Verification items for the finished model (mm, model axes). Give positions to 0.01 mm unless a question says otherwise; leave off trailing zeros. Write each loop counter-clockwise with the first axis right and the second up, starting at its lowest first coordinate (ties: lowest second). Pieces come first, ordered by that corner, then holes.
from build123d import *

# Parameters (mm, degrees)
SKETCH_1_W          = 8
SKETCH_1_H          = 8
EXTRUDE_1_DEPTH     = 20
SKETCH_3_R          = 1.5
CUT_EXTRUDE_1_DEPTH = 23.978250586
SKETCH_5_R          = 1.5
CUT_EXTRUDE_2_DEPTH = 23.978250586


with BuildPart() as part:
    # 草图1 → 凸台-拉伸1 (new body)
    with BuildSketch(Plane(origin=(0, 0, 0), x_dir=(0, 0, -1), z_dir=(1, 0, 0))):
        with Locations((4, 4)):
            Rectangle(SKETCH_1_W, SKETCH_1_H)
    extrude(amount=EXTRUDE_1_DEPTH)

    # 草图3 → 切除-拉伸1 (cut, through all)
    with BuildSketch(Plane.XY):
        with Locations((4, 4)):
            Circle(SKETCH_3_R)
        with Locations((16, 4)):
            Circle(SKETCH_3_R)
    extrude(amount=-CUT_EXTRUDE_1_DEPTH, mode=Mode.SUBTRACT)

    # 草图5 → 切除-拉伸2 (cut, through all)
    with BuildSketch(Plane(origin=(0, 8, 0), x_dir=(1, 0, 0), z_dir=(0, 1, 0))):
        with Locations(Location((10, 4, 0), (0, 0, 270))):
            Circle(SKETCH_5_R)
    extrude(amount=-CUT_EXTRUDE_2_DEPTH, mode=Mode.SUBTRACT)


solid = part.part
Item 1: Depth check by flat-ended pin: pin 1 (1.5 mm diameter, centred on x = 8, z = -6.5, fed in from -Y); pin 2 (1.8 mm diameter, centred on x = 16, y = 4, fed in from -Z). Enter the tip coordinate at first touch or a pass-through.
Answer key:
pin 1: stops at y = 0
pin 2: passes through
Item 2: Sectioned sample at D-D on z = -2.25. Record the cut outline in (x, y).
Answer key:
outline: (0, 0) - (20, 0) - (20, 8) - (0, 8) - close; hole circle Ø3 at (4, 4); hole circle Ø3 at (16, 4)
Item 3: Scan lines: line 1 along Y through (x, z) = (16, -3.5); line 2 along X through (y, z) = (2, -4); line 3 along X through (y, z) = (5.25, -0.25). Record each from-to range of solid material in increasing order.
Answer key:
line 1: y = 0 to 2.5, 5.5 to 8
line 2: x = 0 to 8.5, 11.5 to 20
line 3: x = 0 to 3.17, 4.83 to 15.17, 16.83 to 20
Item 4: Release check for a two-part mould opening along Y. For faces 1 (the face through (10, 0, -6)), 2 (the face through (5.43, 4.45, -3.94)), 3 (the face through (8.67, 4.06, -3.31)), 4 (the face through (14.5, 4.07, -3.94)) record: released by +Y, released by -Y, zero draft, split by the parting line, or undercut.
Answer key:
face 1: released by -Y
face 2: undercut
face 3: zero draft
face 4: undercut
Item 5: Sectioned sample at B-B on y = 4. Record the cut outline in (x, z), then the cut area to 3 significant figures.
Answer key:
outline: (0, -8) - (2.5, -8) - (2.5, 0) - (0, 0) - close; (5.5, -8) - (14.5, -8) - (14.5, 0) - (5.5, 0) - close; (17.5, -8) - (20, -8) - (20, 0) - (17.5, 0) - close; hole circle Ø3 at (10, -4)
area: 105 mm2
Item 6: Sectioned sample at A-A on z = -4. Record the cut outline in (x, y).
Answer key:
outline: (0, 0) - (8.5, 0) - (8.5, 8) - (0, 8) - close; (11.5, 0) - (20, 0) - (20, 8) - (11.5, 8) - close; hole circle Ø3 at (4, 4); hole circle Ø3 at (16, 4)
Item 7: Sectioned sample at C-C on x = 4. Record the cut outline in (y, z).
Answer key:
outline: (0, -8) - (2.5, -8) - (2.5, 0) - (0, 0) - close; (5.5, -8) - (8, -8) - (8, 0) - (5.5, 0) - close
